Source: CAD feature listing. Evaluate the final solid. Frame: model axes, mm. A direction names the side the tool comes from. Give positions to 0.01 mm unless a question says otherwise; leave off trailing zeros. Order: outer loops, then holes, each group sorted by start corner. A loop starts at its lowest first (then second) coordinate and runs counter-clockwise, first axis right, second up.
Autodesk Inventor part; units mm, degrees
ref_plane "YZ Plane" through (0, 0, 0) normal (1, 0, 0) x (0, 1, 0)
ref_plane "XZ Plane" through (0, 0, 0) normal (0, 1, 0) x (-1, 0, 0)
ref_plane "XY Plane" through (0, 0, 0) normal (0, 0, 1) x (1, 0, 0)
sketch "スケッチ1" plane through (0, 0, 0) normal (0, 0, 1) x (1, 0, 0)
  line L0 (0, 0) -> (30, 0)
  line L1 (30, 0) -> (30, 5)
  line L2 (30, 5) -> (5, 30)
  line L3 (5, 30) -> (0, 30)
  line L4 (0, 30) -> (0, 0)
  dimension "d0" = 30
  dimension "d1" = 30
  dimension "d2" = 5
extrude "押し出し1" add sketch "スケッチ1" along normal blind 20
sketch "スケッチ2" plane through (30, 0, 0) normal (1, 0, 0) x (0, 0, -1)
  line L0 (0, 30) -> (-20, 30)
  line L1 (-17.2, 30) -> (-2.8, 30)
  line L2 (-2.8, 30) -> (-2.8, 4)
  line L3 (-2.8, 4) -> (-17.2, 4)
  line L4 (-17.2, 4) -> (-17.2, 30)
  line L5 (0, 0) -> (-20, 0)
  line L6 (0, 30) -> (0, 0)
  line L7 (-20, 5) -> (-20, 30)
  dimension "d5" = 4
  dimension "d6" = 2.8
  dimension "d7" = 2.8
extrude "押し出し2" cut sketch "スケッチ2" against normal blind 26
properties part number "ブラケット2"
1) Ray query, L1, parallel to Z at x = 21.5, y = 12.5; L2, parallel to X at y = 10, z = 14. Return the intervals inside material, ascending.
Checks:
L1: z = 0 to 2.8, 17.2 to 20
L2: x = 0 to 4
2) Section query A-A on x = 8. Output: boundary loops of the cut face in (y, z).
Checks:
outline: (0, 0) - (27, 0) - (27, 2.8) - (4, 2.8) - (4, 17.2) - (27, 17.2) - (27, 20) - (0, 20) - close
3) First-contact query: pin 1 Ø11.5 at (x, z) = (17, 9.5) entering from +Y; pin 2 Ø4 at (x, y) = (23.5, 16) entering from +Z; pin 3 Ø3 at (x, z) = (14, 16.5) entering from +Y; pin 4 Ø6 at (x, z) = (9, 3.5) entering from +Y. Flat tips, straight axial feed; report the tip coordinate or a pass-through.
Checks:
pin 1: stops at y = 4
pin 2: passes through
pin 3: stops at y = 22.33
pin 4: stops at y = 28.92
4) Reachability of faces 1 (the face through (0, 15, 10)), 2 (the face through (4, 17, 10)) from +Z, -Z, +X, -X, +Y, -Y: full face, straight path, thin tool, end or side. Return the list, or none.
Checks:
face 1: +Z, -Z, -X, +Y, -Y
face 2: +X, +Y
5) Section query C-C on z = 12.5. Output: boundary loops of the cut face in (x, y), and give its area (3 significant figures).
Checks:
outline: (0, 0) - (30, 0) - (30, 4) - (4, 4) - (4, 30) - (0, 30) - close
area: 224 mm2
6) Section query B-B on y = 17.5. Output: boundary loops of the cut face in (x, z).
Checks:
outline: (0, 0) - (17.5, 0) - (17.5, 2.8) - (4, 2.8) - (4, 17.2) - (17.5, 17.2) - (17.5, 20) - (0, 20) - close
